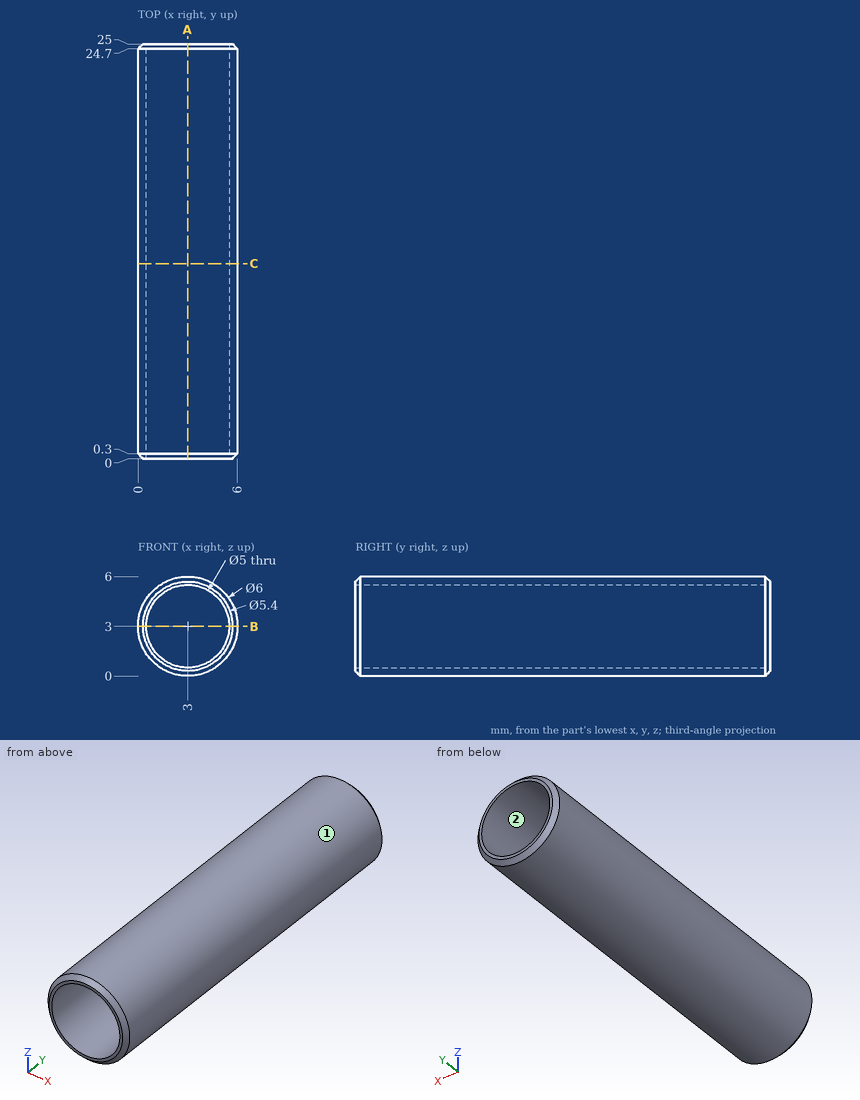
Study the drawing (mm; zero at the part's minimum x, y, z) and answer. Give positions to 0.01 mm unless a question says otherwise; leave off trailing zeros. Write each loop counter-clockwise with the first axis right and the second up, starting at its lowest first coordinate (ties: lowest second). Pieces come first, ordered by that corner, then holes. Notation, with made-up numbers: (63.5, 13.25) -> (118.5, 13.25) arc R14 ccw to (118.5, 30.25) -> close; hole circle Ø4 at (82.25, -8.5). An arc over 180 degrees is marked (long way). Answer in a Markdown table with one row per item.
1) Section C-C on y = 11.75 is taken. Give the vertices of the cut face in (x, z).
Results list:
| item | result |
|---|---|
| outline | circle Ø6 at (3, 3); hole circle Ø5 at (3, 3) |
2) This flat-tipped pin is pushed along its axis until it touches: pin 1 Ø1 at (x, y) = (1, 4) entering from -Z. Where does it stop, or does it pass through?
Results list:
| item | result |
|---|---|
| pin 1 | z = 0.4 |
3) Section B-B on z = 3 is taken. Give the vertices of the cut face in (x, y), plus the area to 3 significant figures.
Results list:
| item | result |
|---|---|
| outline | (0, 0.3) -> (0.3, 0) -> (0.5, 0) -> (0.5, 25) -> (0.3, 25) -> (0, 24.7) -> close; (5.5, 0) -> (5.7, 0) -> (6, 0.3) -> (6, 24.7) -> (5.7, 25) -> (5.5, 25) -> close |
| area | 24.8 mm^2 |
4) Section A-A on x = 3 is taken. Give the vertices of the cut face in (y, z), plus the area to 3 significant figures.
Results list:
| item | result |
|---|---|
| outline | (0, 0.3) -> (0.3, 0) -> (24.7, 0) -> (25, 0.3) -> (25, 0.5) -> (0, 0.5) -> close; (0, 5.5) -> (25, 5.5) -> (25, 5.7) -> (24.7, 6) -> (0.3, 6) -> (0, 5.7) -> close |
| area | 24.8 mm^2 |
5) Determine the mould class of the marked faces 1 and 2 for opening direction X: released by +X, released by -X, zero draft, split by the parting line, or undercut.
Results list:
| item | result |
|---|---|
| face 1 | split by the parting line |
| face 2 | undercut |
6) Straight lines are drawn through the part: line 1 (Z direction, x = 3, y = 17.5); line 2 (X direction, y = 12.5, z = 5); line 3 (X direction, y = 8.5, z = 2.2). For each, find the intervals that lie inside material, in ascending order. Write a range as [from, to].
Results list:
| item | result |
|---|---|
| line 1 | [0, 0.5], [5.5, 6] |
| line 2 | [0.76, 1.5], [4.5, 5.24] |
| line 3 | [0.11, 0.63], [5.37, 5.89] |
